Part print with two shaded views. Sizes in mm from the minimum x, y, z corner. Round coordinates to 2 decimals unless told otherwise and drop trailing zeros. Order: outer loops, then holes, each group sorted by start corner. A loop starts at its lowest first (then second) coordinate and runs counter-clockwise, first axis right, second up. Notation, with made-up numbers: (39.25, 15.25) -> (87.25, 15.25) arc R20 ccw to (87.25, 38.25) -> close; hole circle Ø2 at (15.25, -17.5). An arc over 180 degrees is marked (long way). Use a Markdown table: item, result. Add a question column.
Item 1: Slice it at A-A, the plane y = 140. Give the cut face in (x, z).
Item 2: Probe L1, parallel to X at y = 205, z = 10.25; L2, parallel to X at y = 206, z = 10.75. List the from-to ranges inside material, lowest first.
Item 3: Pin check, flat tips, straight feed: pin 1 (12 mm diameter, centred on x = 265, z = 8.5, fed in from -Y); pin 2 (8 mm diameter, centred on x = 29.78, y = 140, fed in from -Z). Stop position of each tip, or through.
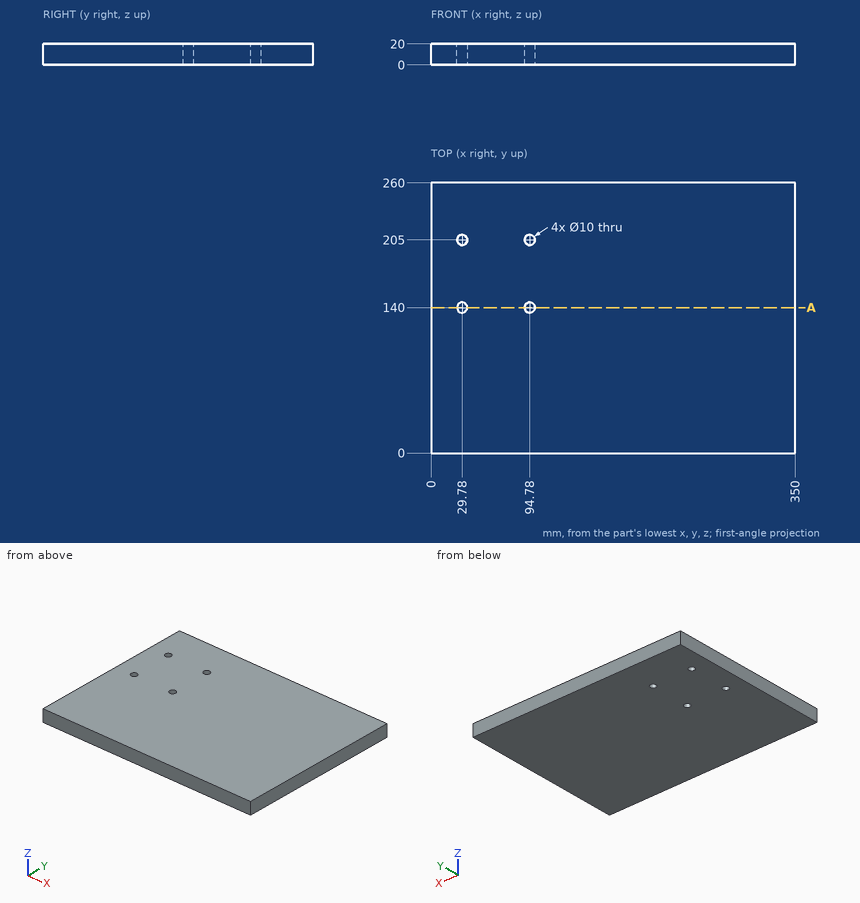
Check sheet entries:
| question | item | result |
|---|---|---|
| 1 | outline | (0, 0) -> (24.78, 0) -> (24.78, 20) -> (0, 20) -> close; (34.78, 0) -> (89.78, 0) -> (89.78, 20) -> (34.78, 20) -> close; (99.78, 0) -> (350, 0) -> (350, 20) -> (99.78, 20) -> close |
| 2 | L1 | 0 to 24.78, 34.78 to 89.78, 99.78 to 350 |
| 2 | L2 | 0 to 24.88, 34.68 to 89.88, 99.68 to 350 |
| 3 | pin 1 | y = 0 |
| 3 | pin 2 | through |
